```python
from build123d import *

# Parameters (mm, degrees)
EXTRUDE1_DEPTH     = 100
SKETCH2_R          = 30
CUT_EXTRUDE1_DEPTH = 1
SKETCH3_W          = 40
SKETCH3_H          = 20
EXTRUDE2_DEPTH     = 40
SKETCH4_W          = 100
SKETCH4_H          = 60
EXTRUDE3_DEPTH     = 1


with BuildPart() as part:
    # Sketch1 → Extrude1 (new body)
    with BuildSketch(Plane(origin=(0, 0, 0), x_dir=(0, 0, -1), z_dir=(1, 0, 0))):
        Polygon((100, 0), (0, 0), (0, 80), (60, 80), align=None)
    extrude(amount=EXTRUDE1_DEPTH)

    # Sketch2 → Cut-Extrude1 (cut)
    with BuildSketch(Plane.XY):
        with Locations((50, 40)):
            Circle(SKETCH2_R)
    extrude(amount=-CUT_EXTRUDE1_DEPTH, mode=Mode.SUBTRACT)

    # Sketch3 → Extrude2 (add)
    with BuildSketch(Plane(origin=(0, 80, 0), x_dir=(-1, 0, 0), z_dir=(0, 1, 0))):
        with Locations((-50, -30)):
            Rectangle(SKETCH3_W, SKETCH3_H)
    extrude(amount=EXTRUDE2_DEPTH)

    # Sketch4 → Extrude3 (add)
    with BuildSketch(Plane(origin=(0, 120, 0), x_dir=(-1, 0, 0), z_dir=(0, 1, 0))):
        with Locations((-50, -30)):
            Rectangle(SKETCH4_W, SKETCH4_H)
    extrude(amount=EXTRUDE3_DEPTH)


solid = part.part
```
Source: CAD feature listing. Evaluate the final solid. Frame: model axes, mm. A direction names the side the tool comes from. Round coordinates to 2 decimals unless told otherwise and drop trailing zeros. Loops run counter-clockwise (first coordinate to the right, second up) from the corner with the lowest first, then second, coordinate; pieces in that order, holes last.
(1) Pull-direction query (Y, two-part tool) for faces 1 (the flat face through (49, 80, -16)), 2 (the flat face through (51, 121, -30)), 3 (the flat face through (100, 41, -40)); classes: +Y half, -Y half, draft (parallel to the pull), parting line (faces both ways), or undercut.
From the geometry:
face 1: undercut
face 2: +Y half
face 3: draft
(2) Section query A-A (x = 88). Output: boundary loops of the cut face in (y, z).
From the geometry:
outline: (0, -100) - (80, -60) - (80, 0) - (0, 0) - close; (120, -60) - (121, -60) - (121, 0) - (120, 0) - close
(3) Section query D-D (x = 74). Output: boundary loops of the cut face in (y, z).
From the geometry:
outline: (0, -100) - (80, -60) - (80, 0) - (58, 0) - (58, -1) - (22, -1) - (22, 0) - (0, 0) - close; (120, -60) - (121, -60) - (121, 0) - (120, 0) - close
(4) Section query B-B (y = 40). Output: boundary loops of the cut face in (x, z).
From the geometry:
outline: (0, -80) - (100, -80) - (100, 0) - (80, 0) - (80, -1) - (20, -1) - (20, 0) - (0, 0) - close
(5) Access query for faces 4 (the flat face through (50, 100, -20)), 5 (the cylindrical face through (43.497, 10.713, -0.493)), 6 (the flat face through (51, 120, -16)), 7 (the flat face through (70, 100, -30)). Directions: +Z, -Z, +X, -X, +Y, -Y. A direction counts if a zero-diameter tool reaches every point of the face in a straight line with its end or side. Return the directions, or none.
From the geometry:
face 4: +Z, +X, -X
face 5: +Z
face 6: none
face 7: +Z, -Z, +X
(6) Material intervals for probe 1 along Y at (x, z) = (50, -0.75); probe 2 along Y at (x, z) = (16.5, -19); probe 3 along X at (y, z) = (82.5, -28), sorted ascending.
From the geometry:
probe 1: y = 0 to 10, 70 to 80, 120 to 121
probe 2: y = 0 to 80, 120 to 121
probe 3: x = 30 to 70
(7) Section query C-C (z = -83). Output: boundary loops of the cut face in (x, y), and give its area (3 significant figures).
From the geometry:
outline: (0, 0) - (100, 0) - (100, 34) - (0, 34) - close
area: 3,400 mm2
(8) Contact query for flat-ended pins moving along their axis: pin 1 Ø12 at (x, y) = (86.5, 38) entering from -Z; pin 2 Ø1.1 at (x, y) = (56, 120.5) entering from -Z; pin 3 Ø18 at (x, y) = (41.5, 31.5) entering from +Z; pin 4 Ø12 at (y, z) = (64, -75) entering from +X. Output: stop coordinate, or through.
From the geometry:
pin 1: stops at z = -84
pin 2: stops at z = -60
pin 3: stops at z = -1
pin 4: passes through
